For this review, take the finished solid that the model builds, in its own axes (mm). Face numbers are marked on the shaded views. A direction names the side the tool comes from. Round coordinates to 2 decimals unless told otherwise and drop trailing zeros. Write each loop counter-clockwise with the first axis right and the second up, starting at its lowest first coordinate (ties: lowest second). Pieces come first, ordered by that corner, then holes. Notation, with made-up numbers: (85, 14.25) - (115, 14.25) arc R18 cw to (115, 35.25) - close; hole circle Ø4 at (87, 37.25). An arc over 180 degrees is marked (long way). One line per item, written item: value. Start each with the question number.
Q1. Mouldability with a two-part tool opening along Y and no side actions: class the marked faces 1, 2 and 3 as +Y half, -Y half, draft (parallel to the pull), parting line (faces both ways), or undercut.
Q2. Add section C-C on x = 15. Write out the cut boundary in (y, z).
Q3. For probe 1 along X at (y, z) = (13.5, 5.5); probe 2 along X at (y, z) = (6.5, 4.25); probe 3 along X at (y, z) = (14, 9.25), list the stretches that pass through material, from the lowest coordinate up.
Q4. Tool access review of the marked faces 4 and 5: name each direction out of +Z, -Z, +X, -X, +Y, -Y from which nothing blocks a thin tool from reaching the whole face with its end or side.
Q5. Add section A-A on x = -15. Write out the cut boundary in (y, z), and give its area (3 significant figures).
Q6. Add section D-D on z = 5. Write out the cut boundary in (x, y), and give its area (3 significant figures).
Q7. Add section B-B on y = 0. Write out the cut boundary in (x, z), and give its area (3 significant figures).
Q8. Clearance check with a flat-ended pin moving along its axis: pin 1 Ø2 at (x, y) = (8.5, -18) entering from -Z. State where the tip first meets the part, or that it passes through.
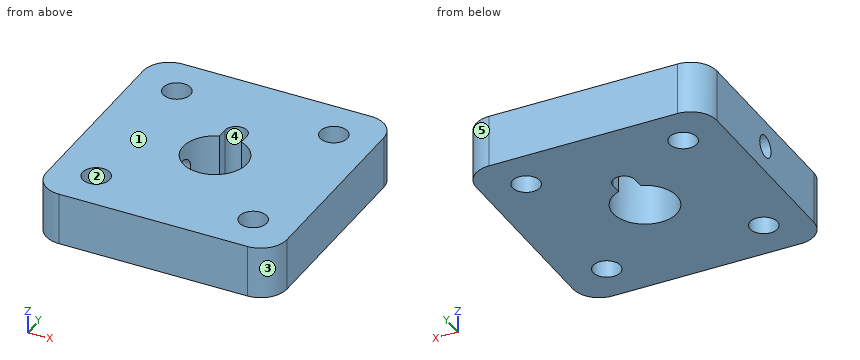
Autodesk Inventor part; units mm, degrees
ref_plane "YZ Plane" through (0, 0, 0) normal (1, 0, 0) x (0, 1, 0)
ref_plane "XZ Plane" through (0, 0, 0) normal (0, 1, 0) x (-1, 0, 0)
ref_plane "XY Plane" through (0, 0, 0) normal (0, 0, 1) x (1, 0, 0)
sketch "スケッチ1" plane through (0, 0, 0) normal (0, 0, 1) x (1, 0, 0)
  circle A0 centre (0, 0) radius 6.1
  circle A1 centre (0, 0) radius 21.2132 construction
  line L0 (0, 0) -> (15, 15) construction
  line L1 (0, 0) -> (0, 37.5908) construction
  circle A2 centre (15, 15) radius 2.6
  circle A3 centre (-15, 15) radius 2.6
  circle A4 centre (-15, -15) radius 2.6
  circle A5 centre (15, -15) radius 2.6
  line L2 (-15, 15) -> (15, 15) construction
  line L3 (15, 15) -> (15, -15) construction
  line L4 (15, -15) -> (-15, -15) construction
  line L5 (-15, -15) -> (-15, 15) construction
  line L6 (-23, -23) -> (23, -23)
  line L7 (23, -23) -> (23, 23)
  line L8 (23, 23) -> (-23, 23)
  line L9 (-23, 23) -> (-23, -23)
  line L10 (-23, -23) -> (23, 23) construction
  line L11 (23, -23) -> (-23, 23) construction
  circle A6 centre (0, 0) radius 15 construction
  circle A7 centre (-15, 15) radius 5.7791 construction
  dimension "d1" = 12.2
  dimension "d3" = 45
  dimension "d4" = 5.2
  dimension "d7" = 360
  dimension "d11" = 30
  dimension "d12" = 46
extrude "押し出し1" add sketch "スケッチ1" along normal blind 10
sketch "スケッチ2" plane through (-23, -23, 0) normal (-1, 0, 0) x (0, 0, 1)
  line L0 (0, 23) -> (10, 23) construction
  line L1 (10, 29.1) -> (10, 16.9) construction
  circle A0 centre (5, 23) radius 2.1
  dimension "d14" = 4.2
extrude "押し出し2" cut sketch "スケッチ2" against normal up to next
fillet "フィレット2" radius 5 4 edges at (23, -23, 5) (23, 23, 5) (-23, -23, 5) (-23, 23, 5)
sketch "スケッチ3" plane through (0, 0, 10) normal (0, 0, 1) x (1, 0, 0)
  circle A0 centre (0, 0) radius 6.1
  line L0 (-2.1, 5.7271) -> (-2.1, 7.8)
  line L1 (-2.1, 7.8) -> (2.1, 7.8) construction
  line L2 (2.1, 7.8) -> (2.1, 5.7271)
  line L3 (0, 0) -> (0, 23) construction
  line L4 (18, 23) -> (-18, 23) construction
  arc A1 (2.1, 7.8) -> (-2.1, 7.8) centre (0, 7.8) ccw
  line L5 (-2.1, 5.7271) -> (2.1, 5.7271)
  point P0 (0, 6.1)
  dimension "d18" = 2.1
  dimension "d23" = 7.8
extrude "押し出し3" cut sketch "スケッチ3" against normal blind 10 contours A0 L0 A1 L2
properties part number "車輪ハブ3"
Result set:
1. face 1: draft
1. face 2: undercut
1. face 3: -Y half
2. outline: (-23, 0) - (-17.6, 0) - (-17.6, 10) - (-23, 10) - close; (-12.4, 0) - (12.4, 0) - (12.4, 10) - (-12.4, 10) - close; (17.6, 0) - (23, 0) - (23, 10) - (17.6, 10) - close
3. probe 1: x = -23 to -17.12, -12.88 to 12.88, 17.12 to 23
3. probe 2: x = -23 to -2.1, 2.1 to 23
3. probe 3: x = -23 to -17.4, -12.6 to 12.6, 17.4 to 23
4. face 4: +Z, -Z
4. face 5: +Z, -Z, +X, +Y
5. outline: (-23, 0) - (-17.6, 0) - (-17.6, 10) - (-23, 10) - close; (-12.4, 0) - (12.4, 0) - (12.4, 10) - (-12.4, 10) - close; (17.6, 0) - (23, 0) - (23, 10) - (17.6, 10) - close; hole circle Ø4.2 at (0, 5)
5. area: 342 mm^2
6. outline: (-23, -18) arc R5 ccw to (-18, -23) - (18, -23) arc R5 ccw to (23, -18) - (23, 18) arc R5 ccw to (18, 23) - (-18, 23) arc R5 ccw to (-23, 18) - (-23, 2.1) - (-5.73, 2.1) arc R6.1 cw to (-2.1, 5.73) - (-2.1, 7.8) arc R2.1 cw to (2.1, 7.8) - (2.1, 5.73) arc R6.1 cw (long way) to (-5.73, -2.1) - (-23, -2.1) - close; hole circle Ø5.2 at (-15, -15); hole circle Ø5.2 at (-15, 15); hole circle Ø5.2 at (15, -15); hole circle Ø5.2 at (15, 15)
6. area: 1,810 mm^2
7. outline: (-23, 0) - (-6.1, 0) - (-6.1, 2.9) - (-23, 2.9) - close; (-23, 7.1) - (-6.1, 7.1) - (-6.1, 10) - (-23, 10) - close; (6.1, 0) - (23, 0) - (23, 10) - (6.1, 10) - close
7. area: 267 mm^2
8. pin 1: stops at z = 0
